from build123d import *

# Parameters (mm, degrees)
F1_DEPTH = 31.75
F2_R     = 7.0115347254
F3_DEPTH = 31.751
F4_W     = 78.8504332304
F4_H     = 27.2497832775
F5_DEPTH = 33.274
F7_DEPTH = 33.9844357044


# Not quite as in the source:
# - a feature of the source that left no trace in its solid (it failed there, or was rolled back) is left out


with BuildPart() as f1:
    # F0 (on Top) → F1 (new body)
    with BuildSketch(Plane.XY):
        with BuildLine():
            Line((39.576777419, 20.2923920006), (-39.5247050543, 20.2923920006))
            ThreePointArc((-39.5247050543, 20.2923920006), (-26.2003502762, 13.8037157784), (-20.8060217658, 0))
            ThreePointArc((-20.8060217658, 0), (-26.2003502762, -13.8037157784), (-39.5247050543, -20.2923920006))
            Line((-39.5247050543, -20.2923920006), (39.576777419, -20.2923920006))
            ThreePointArc((39.576777419, -20.2923920006), (20.8101499679, 0), (39.576777419, 20.2923920006))
        make_face()
        with BuildLine():
            Line((-39.5247050543, 20.2923920006), (-41.1645658314, 20.2923920006))
            Line((-41.1645658314, 20.2923920006), (-41.1645658314, -20.2923920006))
            Line((-41.1645658314, -20.2923920006), (-39.5247050543, -20.2923920006))
            ThreePointArc((-39.5247050543, -20.2923920006), (-26.2003502762, -13.8037157784), (-20.8060217658, 0))
            ThreePointArc((-20.8060217658, 0), (-26.2003502762, 13.8037157784), (-39.5247050543, 20.2923920006))
        make_face()
        with BuildLine():
            Line((-41.1645658314, -20.2923920006), (-41.1645658314, 20.2923920006))
            Line((-41.1645658314, 20.2923920006), (-39.5247050543, 20.2923920006))
            ThreePointArc((-39.5247050543, 20.2923920006), (-61.5231098971, 0), (-39.5247050543, -20.2923920006))
            Line((-39.5247050543, -20.2923920006), (-41.1645658314, -20.2923920006))
        make_face()
        with BuildLine():
            Line((41.1645658314, 20.2923920006), (39.576777419, 20.2923920006))
            ThreePointArc((39.576777419, 20.2923920006), (20.8101499679, 0), (39.576777419, -20.2923920006))
            Line((39.576777419, -20.2923920006), (41.1645658314, -20.2923920006))
            Line((41.1645658314, -20.2923920006), (41.1645658314, 20.2923920006))
        make_face()
        with BuildLine():
            ThreePointArc((61.518981695, 0), (54.9845466472, 14.9435730466), (39.576777419, 20.2923920006))
            Line((39.576777419, 20.2923920006), (41.1645658314, 20.2923920006))
            Line((41.1645658314, 20.2923920006), (41.1645658314, -20.2923920006))
            Line((41.1645658314, -20.2923920006), (39.576777419, -20.2923920006))
            ThreePointArc((39.576777419, -20.2923920006), (54.9845466472, -14.9435730466), (61.518981695, 0))
        make_face()
    extrude(amount=F1_DEPTH)

    # F2 (on face) → F3 (cut, through all)
    with BuildSketch(Plane.XY.offset(31.75)):
        with Locations((50.1511953771, 0)):
            Circle(F2_R)
        with Locations((-50.1511953771, 0)):
            Circle(F2_R)
    extrude(amount=-F3_DEPTH, mode=Mode.SUBTRACT)

    # F4 (on face) → F5 (join)
    with BuildSketch(Plane.XY.offset(31.75)):
        Rectangle(F4_W, F4_H)
    extrude(amount=F5_DEPTH)

    # F6 (on face) → F7 (cut, through all)
    with BuildSketch(Plane.XZ.offset(13.6248916388)):
        with BuildLine():
            ThreePointArc((-25.020677247, 65.024), (0, 40.003322753), (25.020677247, 65.024))
            Line((25.020677247, 65.024), (-25.020677247, 65.024))
        make_face()
    extrude(amount=-F7_DEPTH, mode=Mode.SUBTRACT)


solid = f1.part
Model file for the job. Use its own axes, mm. A direction names the side the tool comes from. Give positions to 0.01 mm unless a question says otherwise; leave off trailing zeros. Order: outer loops, then holes, each group sorted by start corner. A loop starts at its lowest first (then second) coordinate and runs counter-clockwise, first axis right, second up. Notation, with made-up numbers: M -34,54 L -7,54 A25 cw -7,89 Z; hole C -25,73.5 d10. An arc over 180 degrees is marked long. Write item = value, one per line.
Q1. Cut at C-C, the plane x = 0. List the corners of the cut face in (y, z), then the cut area to 3 significant figures.
Derived:
outline = M -20.29,0 L 20.29,0 L 20.29,31.75 L 13.62,31.75 L 13.62,40 L -13.62,40 L -13.62,31.75 L -20.29,31.75 Z
area = 1,510 mm2
Q2. Cut at A-A, the plane z = 10.5. List the corners of the cut face in (x, y).
Derived:
outline = M -39.52,-20.29 L 39.58,-20.29 A20.35 ccw long 39.58,20.29 L -39.52,20.29 A20.36 ccw long Z; hole C -50.15,0 d14.02; hole C 50.15,0 d14.02
Q3. Drill centre lines: line 1 (X direction, y = -5.5, z = 5); line 2 (Y direction, x = 20.5, z = 5.5); line 3 (X direction, y = -2, z = 25.5). Where is each one in solid material? Low to high. Write a range as [from, to].
Derived:
line_1 = [-60.77, -54.5], [-45.8, 45.8], [54.5, 60.76]
line_2 = [-20.29, 20.29]
line_3 = [-61.42, -56.87], [-43.43, 43.43], [56.87, 61.42]
Q4. Tool access for faces 4 (the flat face through (-1, -13.625, 37)), 5 (the flat face through (-39.425, 0, 48)), 6 (the flat face through (-1, 13.625, 37)): list every direction of +Z, -Z, +X, -X, +Y, -Y with a clear straight run to the whole face (end or side of a thin tool).
Derived:
face_4 = +Z, +X, -X, -Y
face_5 = +Z, -X, +Y, -Y
face_6 = +Z, +X, -X, +Y
Q5. Cut at D-D, the plane z = 53. List the corners of the cut face in (x, y).
Derived:
outline = M -39.43,-13.62 L -21.94,-13.62 L -21.94,13.62 L -39.43,13.62 Z; M 21.94,-13.62 L 39.43,-13.62 L 39.43,13.62 L 21.94,13.62 Z
Q6. Two-plate mould, pull along X, no slides. Class faces 1 (the flat face through (39.425, 0, 48)), 2 (the cylindrical face through (-0.55, -0.19, 40.01)), 3 (the flat face through (32, 0, 65.024)): pulls with the +X half, pulls with the -X half, needs draft (parallel to the pull), parting line crosses it, or undercut.
Derived:
face_1 = pulls with the +X half
face_2 = undercut
face_3 = needs draft
Q7. Flat gauge pins, fed straight in: pin 1 (10 mm diameter, centred on y = 10.5, z = 53.5, fed in from +X); pin 2 (9.5 mm diameter, centred on x = -17.5, z = 9.5, fed in from +Y); pin 3 (4 mm diameter, centred on x = -31, z = 52.5, fed in from +Y); pin 4 (22.5 mm diameter, centred on x = -50.15, y = 0, fed in from -Z). Where does each tip first touch, or does it go through?
Derived:
pin_1 = 39.43
pin_2 = 20.29
pin_3 = 13.62
pin_4 = 0
Q8. Cut at B-B, the plane y = 5.5. List the corners of the cut face in (x, z).
Derived:
outline = M -60.77,0 L -54.5,0 L -54.5,31.75 L -60.77,31.75 Z; M -45.8,0 L 45.8,0 L 45.8,31.75 L 39.43,31.75 L 39.43,65.02 L 25.02,65.02 A25.02 cw -25.02,65.02 L -39.43,65.02 L -39.43,31.75 L -45.8,31.75 Z; M 54.5,0 L 60.76,0 L 60.76,31.75 L 54.5,31.75 Z
